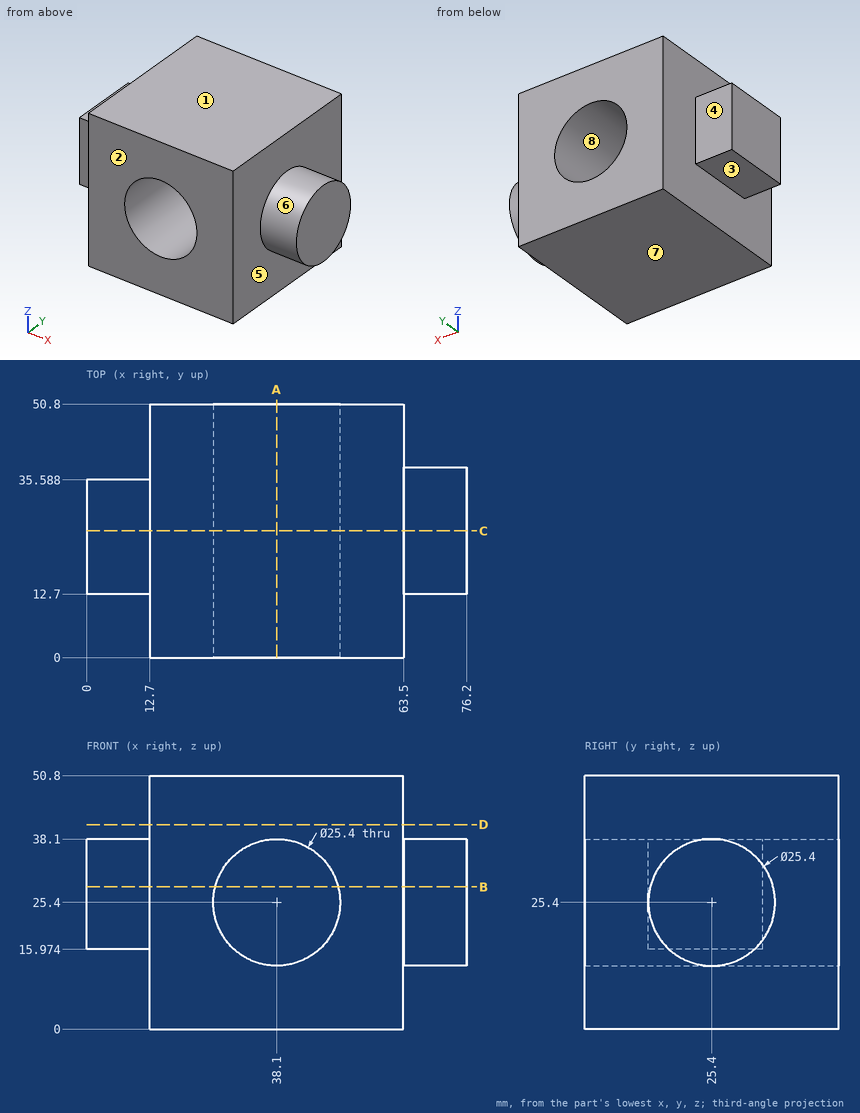
Can you work these out from the drawing? Everything is in mm from the part's minimum corner. A direction names the side the tool comes from. Coordinates: 2 decimals unless noted, no trailing zeros. Loops run counter-clockwise (first coordinate to the right, second up) from the corner with the lowest first, then second, coordinate; pieces in that order, holes last.
1. Imagine slicing it at A-A, the plane x = 38.1. Please give me the cut outline in (y, z).
2. I need wall thicknesses on L1, parallel to Z at x = 37.5, y = 13.5; L2, parallel to X at y = 17.5, z = 15.5 (1 decimal); L3, parallel to X at y = 8.5, z = 21.5. Which ranges of each line are inside material? Lowest first, please.
3. If we mould it in two halves opening along Z, with no side actions, what happens to the marked faces 6, 7 and 8? For each: pulls with the +Z half, pulls with the -Z half, needs draft (parallel to the pull), parting line crosses it, or undercut.
4. Imagine slicing it at D-D, the plane z = 41. Please give me the cut outline in (x, y).
5. Imagine slicing it at C-C, the plane y = 25.4. Please give me the cut outline in (x, z).
6. For the marked faces 1, 2, 3, 4 and 5, which set-ups out of +Z, -Z, +X, -X, +Y, -Y let a thin tool reach every point of the face, with its end or its side?
7. Imagine slicing it at B-B, the plane z = 28.5. Please give me the cut outline in (x, y).
8. For P1, Ø6.5, axis at x = 7.5, z = 24, coming from the +Y side; P2, Ø5, axis at y = 7.5, z = 17.5, coming from the -X side; P3, Ø4, axis at x = 6.5, y = 26.5, coming from the +Z side, each with a flat end and sliding along its axis, tell me the tip position at first contact or that it passes through.
Taken from the geometry:
1. outline: (0, 0) - (50.8, 0) - (50.8, 12.7) - (0, 12.7) - close; (0, 38.1) - (50.8, 38.1) - (50.8, 50.8) - (0, 50.8) - close
2. L1: z = 0 to 12.71, 38.09 to 50.8
2. L2: x = 12.7 to 30.1, 46.1 to 76.2
2. L3: x = 12.7 to 26.01, 50.19 to 63.5
3. face 6: parting line crosses it
3. face 7: pulls with the -Z half
3. face 8: undercut
4. outline: (12.7, 0) - (63.5, 0) - (63.5, 50.8) - (12.7, 50.8) - close
5. outline: (0, 15.97) - (12.7, 15.97) - (12.7, 0) - (63.5, 0) - (63.5, 12.7) - (76.2, 12.7) - (76.2, 38.1) - (63.5, 38.1) - (63.5, 50.8) - (12.7, 50.8) - (12.7, 38.1) - (0, 38.1) - close; hole circle Ø25.4 at (38.1, 25.4)
6. face 1: +Z, +X, -X, +Y, -Y
6. face 2: +Z, -Z, +X, -X, -Y
6. face 3: -Z, -X, +Y, -Y
6. face 4: +Z, -Z, -X, +Y
6. face 5: +X
7. outline: (0, 12.7) - (12.7, 12.7) - (12.7, 0) - (25.78, 0) - (25.78, 50.8) - (12.7, 50.8) - (12.7, 35.59) - (0, 35.59) - close; (50.42, 0) - (63.5, 0) - (63.5, 13.08) - (76.2, 13.08) - (76.2, 37.72) - (63.5, 37.72) - (63.5, 50.8) - (50.42, 50.8) - close
8. P1: stops at y = 35.59
8. P2: stops at x = 12.7
8. P3: stops at z = 38.1
